Input: part model. Units: mm. Frame: model coordinates. Face numbers are marked on the shaded views. A direction names the side the tool comes from. Round coordinates to 2 decimals unless told otherwise and drop trailing zeros. Loops run counter-clockwise (first coordinate to the right, second up) from the corner with the lowest first, then second, coordinate; pieces in that order, holes last.
(1) Cut plane D-D, the plane z = 2.5. Output: boundary loops of the cut face in (x, y), and give its area (3 significant figures).
(2) Draft query along Y for the marked faces 3, 4 and 5. Return one class per face: released by +Y, released by -Y, zero draft, split by the parting line, or undercut.
(3) Access query for the marked faces 1 and 2. Directions: +Z, -Z, +X, -X, +Y, -Y. A direction counts if a zero-diameter tool reaches every point of the face in a straight line with its end or side. Return the directions, or none.
(4) Line query: line 1 (Y direction, x = 41, z = 6); line 2 (X direction, y = 3, z = 3); line 3 (X direction, y = 3, z = 7.25). Output: solid intervals per line, ascending.
(5) Cut plane C-C, the plane x = 41. Output: boundary loops of the cut face in (y, z).
(6) Cut plane B-B, the plane y = 17. Output: boundary loops of the cut face in (x, z), and give its area (3 significant figures).
(7) Cut plane A-A, the plane x = 14.5. Output: boundary loops of the cut face in (y, z), and give its area (3 significant figures).
from build123d import *

# Parameters (mm, degrees)
SKETCH1_W               = 45
SKETCH1_H               = 30.527185319
SKETCH1_W_2             = 25
SKETCH1_H_2             = 25
BOSS_EXTRUDE1_DEPTH     = 10
SKETCH2_W               = 5
SKETCH2_H               = 25
BOSS_EXTRUDE2_DEPTH     = 3
SKETCH3_W               = 5
SKETCH3_H               = 25
BOSS_EXTRUDE3_DEPTH     = 3
SKETCH4_W               = 19
SKETCH4_H               = 5
BOSS_EXTRUDE4_DEPTH     = 3
SKETCH5_W               = 19
SKETCH5_H               = 5
BOSS_EXTRUDE5_DEPTH     = 3
SKETCH6_R               = 1.5
CUT_EXTRUDE1_DEPTH      = 56.289321243
CUT_EXTRUDE2_DEPTH      = 56.289321243
CUT_EXTRUDE2_DEPTH_BACK = 56.289321243
SKETCH7_W               = 2
SKETCH7_H               = 30.527185319


with BuildPart() as part:
    # Sketch1 → Boss-Extrude1 (new body)
    with BuildSketch(Plane.XY):
        with Locations((22.5, 15.26359266)):
            Rectangle(SKETCH1_W, SKETCH1_H)
        with Locations((22.5, 15.26359266)):
            Rectangle(SKETCH1_W_2, SKETCH1_H_2, mode=Mode.SUBTRACT)
    extrude(amount=BOSS_EXTRUDE1_DEPTH)

    # Sketch2 → Boss-Extrude2 (add)
    with BuildSketch(Plane(origin=(10, 0, 0), x_dir=(0, 0, -1), z_dir=(1, 0, 0))):
        with Locations((-7.5, 15.26359266)):
            Rectangle(SKETCH2_W, SKETCH2_H)
    extrude(amount=BOSS_EXTRUDE2_DEPTH)

    # Sketch3 → Boss-Extrude3 (add)
    with BuildSketch(Plane.ZY.offset(-35)):
        with Locations((7.5, 15.26359266)):
            Rectangle(SKETCH3_W, SKETCH3_H)
    extrude(amount=BOSS_EXTRUDE3_DEPTH)

    # Sketch4 → Boss-Extrude4 (add)
    with BuildSketch(Plane.XZ.offset(-27.76359266)):
        with Locations((22.5, 7.5)):
            Rectangle(SKETCH4_W, SKETCH4_H)
    extrude(amount=BOSS_EXTRUDE4_DEPTH)

    # Sketch5 → Boss-Extrude5 (add)
    with BuildSketch(Plane(origin=(0, 2.76359266, 0), x_dir=(1, 0, 0), z_dir=(0, 1, 0))):
        with Locations((22.5, -7.5)):
            Rectangle(SKETCH5_W, SKETCH5_H)
    extrude(amount=BOSS_EXTRUDE5_DEPTH)

    # Sketch6 → Cut-Extrude1 (cut, through all)
    with BuildSketch(Plane.XY.offset(10)):
        with Locations((4, 27.527185319)):
            Circle(SKETCH6_R)
        with Locations((41, 27.527185319)):
            Circle(SKETCH6_R)
        with Locations(Location((41, 3, 0), (0, 0, 180))):
            Circle(SKETCH6_R)
        with Locations(Location((4, 3, 0), (0, 0, 180))):
            Circle(SKETCH6_R)
    extrude(amount=-CUT_EXTRUDE1_DEPTH, mode=Mode.SUBTRACT)

    # Sketch7 → Cut-Extrude2 (cut, two sides: drawn at the far end of the back side and taken through both)
    with BuildSketch(Plane(origin=(45, 0, 0), x_dir=(0, 0, -1), z_dir=(1, 0, 0)).offset(-CUT_EXTRUDE2_DEPTH_BACK)):
        with Locations((-9, 15.26359266)):
            Rectangle(SKETCH7_W, SKETCH7_H)
    extrude(amount=CUT_EXTRUDE2_DEPTH + CUT_EXTRUDE2_DEPTH_BACK, mode=Mode.SUBTRACT)


solid = part.part
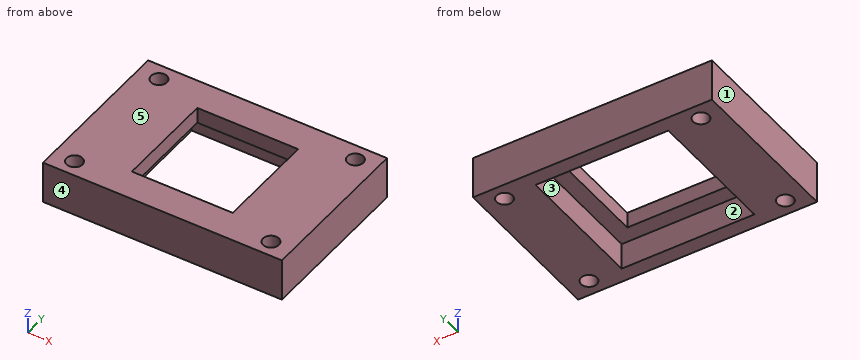
Reported:
1. outline: (0, 0) - (45, 0) - (45, 30.53) - (0, 30.53) - close; hole circle Ø3 at (4, 3); hole circle Ø3 at (4, 27.53); hole (10, 2.76) - (35, 2.76) - (35, 27.76) - (10, 27.76) - close; hole circle Ø3 at (41, 3); hole circle Ø3 at (41, 27.53)
1. area: 720 mm2
2. face 3: undercut
2. face 4: released by -Y
2. face 5: zero draft
3. face 1: +Z, -Z, -X, +Y, -Y
3. face 2: -Z
4. line 1: y = 0 to 1.5, 4.5 to 26.03, 29.03 to 30.53
4. line 2: x = 0 to 2.5, 5.5 to 10, 35 to 39.5, 42.5 to 45
4. line 3: x = 0 to 2.5, 5.5 to 39.5, 42.5 to 45
5. outline: (0, 0) - (1.5, 0) - (1.5, 8) - (0, 8) - close; (4.5, 0) - (26.03, 0) - (26.03, 8) - (4.5, 8) - close; (29.03, 0) - (30.53, 0) - (30.53, 8) - (29.03, 8) - close
6. outline: (0, 0) - (10, 0) - (10, 5) - (13, 5) - (13, 8) - (0, 8) - close; (32, 5) - (35, 5) - (35, 0) - (45, 0) - (45, 8) - (32, 8) - close
6. area: 178 mm2
7. outline: (0, 0) - (2.76, 0) - (2.76, 5) - (5.76, 5) - (5.76, 8) - (0, 8) - close; (24.76, 5) - (27.76, 5) - (27.76, 0) - (30.53, 0) - (30.53, 8) - (24.76, 8) - close
7. area: 62.2 mm2
